Autodesk Inventor part; units mm, degrees
ref_plane "YZ Plane" through (0, 0, 0) normal (1, 0, 0) x (0, 1, 0)
ref_plane "XZ Plane" through (0, 0, 0) normal (0, 1, 0) x (-1, 0, 0)
ref_plane "XY Plane" through (0, 0, 0) normal (0, 0, 1) x (1, 0, 0)
sketch "Sketch1" plane through (0, 0, 0) normal (0, 1, 0) x (-1, 0, 0)
  circle A0 centre (0, 0) radius 5.95
  circle A1 centre (0, -16.35) radius 2.6
  line L0 (4.4, -4.0053) -> (2.5736, -16.7197)
  circle A2 centre (0, 16.35) radius 2.6
  line L1 (4.4, 4.0053) -> (2.5736, 16.7197)
  line L2 (-4.4, 4.0053) -> (-2.6, 16.35)
  line L3 (-4.4, -4.0053) -> (-2.5736, -16.7197)
  dimension "d0" = 11.9
  dimension "d1" = 5.2
  dimension "d2" = 4.4
  dimension "d3" = 5.2
  dimension "d4" = 16.35
  dimension "d5" = 16.35
  dimension "d6" = 4.4
  dimension "d7" = 4.4
  dimension "d8" = 4.4
  dimension "d9" = 0
extrude "Extrusion1" add sketch "Sketch1" along normal blind 2.2
sketch "Sketch2" plane through (0, 0, 0) normal (0, -1, 0) x (1, 0, 0)
  circle A0 centre (0, 0) radius 3.8734
  circle A1 centre (0, 0) radius 3.45
  dimension "d12" = 6.9
extrude "Extrusion2" add sketch "Sketch2" along normal blind 3.2
sketch "Sketch3" plane through (0, 2.2, 0) normal (0, 1, 0) x (1, 0, 0)
  circle A0 centre (0, 0) radius 1.25
  dimension "d15" = 2.5
extrude "Extrusion3" cut sketch "Sketch3" against normal blind 2.2
properties part number "servo_attach"
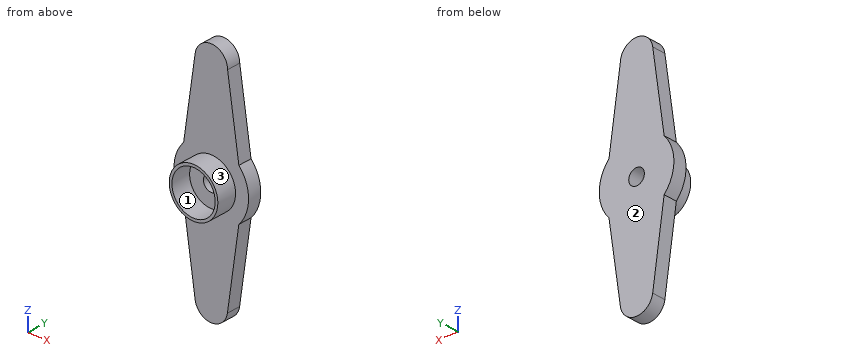
Model file for the job. Use its own axes, mm. Face numbers are marked on the shaded views. Coordinates: 2 decimals unless noted, no trailing zeros. Loops run counter-clockwise (first coordinate to the right, second up) from the corner with the lowest first, then second, coordinate; pieces in that order, holes last. Notation, with made-up numbers: (24.25, 62.5) - (55.25, 62.5) arc R21 ccw to (55.25, 90.5) - close; hole circle Ø11 at (36, -31.5). An arc over 180 degrees is marked (long way). Answer as a JSON object with one key per item and string values. Group by question number.
(1) Flat gauge pins, fed straight in: pin 1 (1 mm diameter, centred on x = 1, z = 0.5, fed in from -Y); pin 2 (1.5 mm diameter, centred on y = -0.5, z = -14.5, fed in from +X); pin 3 (1.5 mm diameter, centred on x = 0, z = 0, fed in from +Y). Where does each tip first touch, or does it go through?
(2) Probe line 1 along X through (y, z) = (1.7, 0); line 2 along Z through (x, y) = (0, -0.95); line 3 along Y through (x, z) = (1.25, 15). List the from-to ranges inside material, lowest first.
(3) Cut at D-D (x = 5.25). Give the cut face in (y, z).
(4) Two-plate mould, pull along X, no slides. Class the marked faces 1, 2 and 3: released by +X, released by -X, zero draft, split by the parting line, or undercut.
(5) Cut at A-A (z = 0). Give the cut face in (x, y).
(6) Cut at C-C (y = 0.65). Give the cut face in (x, z).
(7) Cut at B-B (x = 0). Give the cut face in (y, z), then the cut area to 3 significant figures.
Geometry says:
{
 "1": {"pin 1": "stops at y = 0", "pin 2": "stops at x = 2.97", "pin 3": "passes through"},
 "2": {"line 1": "x = -5.95 to -1.25, 1.25 to 5.95", "line 2": "z = -3.87 to -3.45, 3.45 to 3.87", "line 3": "y = 0 to 2.2"},
 "3": {"outline": "(0, -2.8) - (2.2, -2.8) - (2.2, 2.8) - (0, 2.8) - close"},
 "4": {"face 1": "undercut", "face 2": "zero draft", "face 3": "split by the parting line"},
 "5": {"outline": "(-5.95, 0) - (-3.87, 0) - (-3.87, -3.2) - (-3.45, -3.2) - (-3.45, 0) - (-1.25, 0) - (-1.25, 2.2) - (-5.95, 2.2) - close; (1.25, 0) - (3.45, 0) - (3.45, -3.2) - (3.87, -3.2) - (3.87, 0) - (5.95, 0) - (5.95, 2.2) - (1.25, 2.2) - close"},
 "6": {"outline": "(-4.4, -4.01) - (-2.57, -16.72) arc R2.6 ccw to (2.57, -16.72) - (4.4, -4.01) arc R5.95 ccw to (4.4, 4.01) - (2.6, 16.35) arc R2.6 ccw to (-2.57, 16.72) - (-4.4, 4.01) arc R5.95 ccw to start; hole circle Ø2.5 at (0, 0)"},
 "7": {"outline": "(-3.2, -3.87) - (0, -3.87) - (0, -18.95) - (2.2, -18.95) - (2.2, -1.25) - (0, -1.25) - (0, -3.45) - (-3.2, -3.45) - close; (-3.2, 3.45) - (0, 3.45) - (0, 1.25) - (2.2, 1.25) - (2.2, 18.95) - (0, 18.95) - (0, 3.87) - (-3.2, 3.87) - close", "area": "80.6 mm^2"}
}
